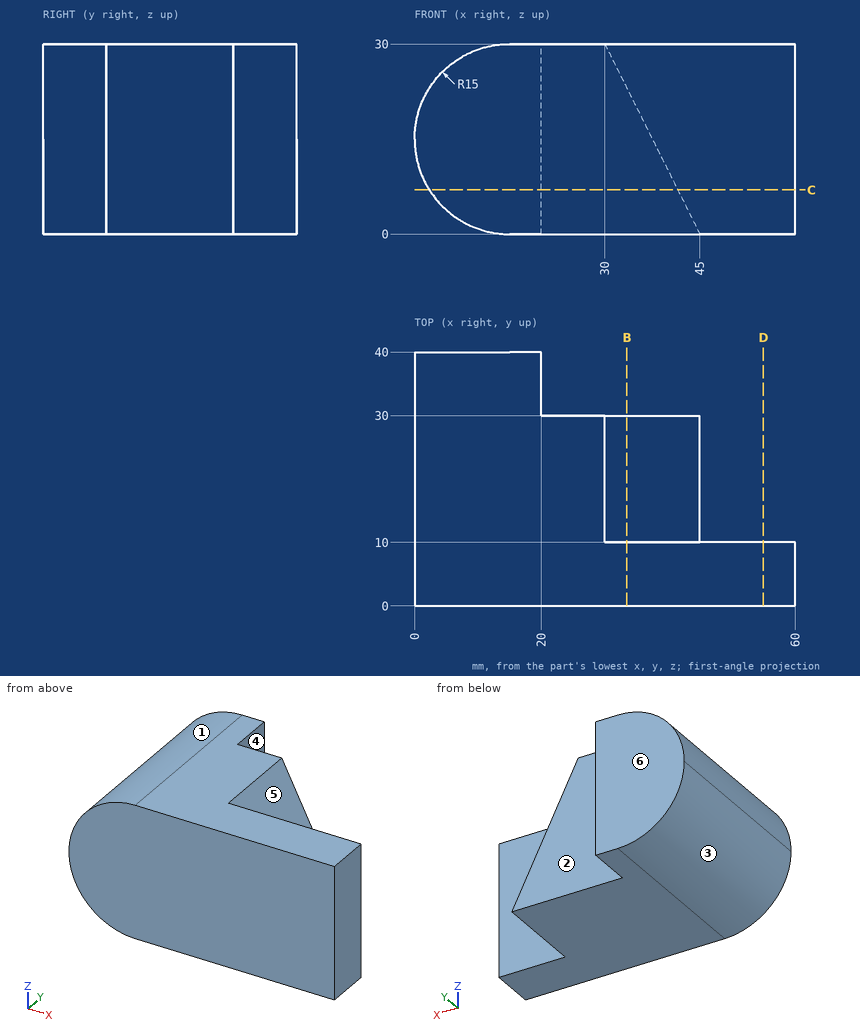
Here's the drawing with two shaded views (mm, measured from the low corner). I have some questions. A direction names the side the tool comes from. Coordinates: 2 decimals unless noted, no trailing zeros. Order: outer loops, then holes, each group sorted by start corner. A loop starts at its lowest first (then second) coordinate and runs counter-clockwise, first axis right, second up.
Item 1: For P1, Ø10, axis at y = 27.5, z = 12, coming from the +X side; P2, Ø2, axis at y = 26, z = 25.5, coming from the -X side; P3, Ø10, axis at x = 44.5, z = 12, coming from the -Y side; P4, Ø1, axis at x = 32.5, y = 15, coming from the +Z side, each with a flat end and sliding along its axis, tell me the tip position at first contact or that it passes through.
Result sheet:
P1: stops at x = 41.5
P2: stops at x = 3.39
P3: stops at y = 0
P4: stops at z = 26
Item 2: If we section it at C-C on z = 7: List the corners of the cut face in (x, y) for me.
Result sheet:
outline: (2.31, 0) - (60, 0) - (60, 10) - (41.5, 10) - (41.5, 30) - (20, 30) - (20, 40) - (2.31, 40) - close
Item 3: For the marked faces 4, 5 and 6, which set-ups out of +Z, -Z, +X, -X, +Y, -Y let a thin tool reach every point of the face, with its end or its side?
Result sheet:
face 4: +Z, -Z, +X, +Y
face 5: +Z, +X, +Y
face 6: +Z, -Z, +X, -X, +Y
Item 4: If we section it at D-D on x = 55: List the corners of the cut face in (y, z) for me, plus the area to 3 significant figures.
Result sheet:
outline: (0, 0) - (10, 0) - (10, 30) - (0, 30) - close
area: 300 mm2
Item 5: If we mould it in two halves opening along Z, with no side actions, what happens to the marked faces 1, 2 and 3? For each: +Z half, -Z half, draft (parallel to the pull), parting line (faces both ways), or undercut.
Result sheet:
face 1: +Z half
face 2: draft
face 3: -Z half
Item 6: I need wall thicknesses on line 1 (Y direction, x = 25.5, z = 19); line 2 (Y direction, x = 47, z = 23); line 3 (Z direction, x = 11.5, y = 29). Which ranges of each line are inside material? Lowest first, please.
Result sheet:
line 1: y = 0 to 30
line 2: y = 0 to 10
line 3: z = 0.41 to 29.59
Item 7: If we section it at B-B on x = 33.5: List the corners of the cut face in (y, z) for me.
Result sheet:
outline: (0, 0) - (30, 0) - (30, 23) - (10, 23) - (10, 30) - (0, 30) - close
